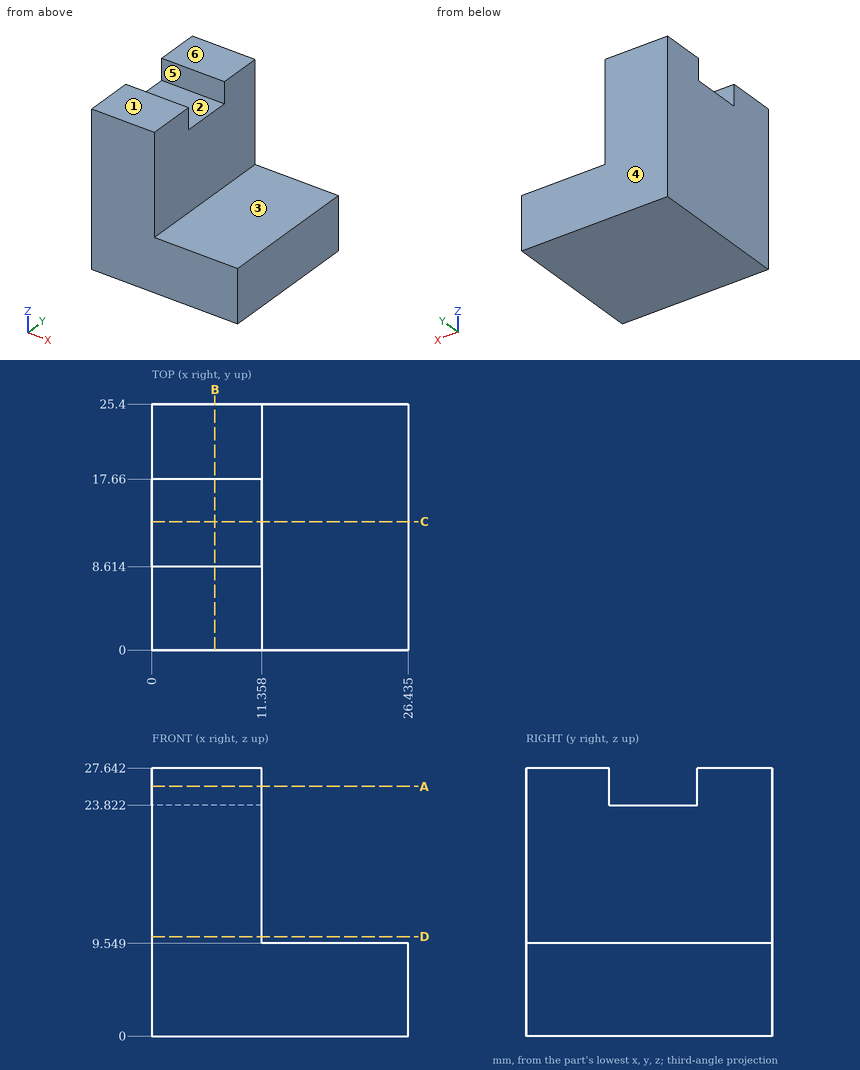
Answer from the drawing. Dimensions are ordinates in mm from the lowest x, y and z of the part. A direction names the side the tool comes from. Coordinates: 2 decimals unless noted, no trailing zeros. Order: outer loops, then holes, each group sorted by start corner. A loop starts at its lowest first (then second) coordinate and runs counter-clockwise, first axis right, second up. Notation, with made-up numbers: M 6.5,88.5 L 44.5,88.5 A26 ccw 44.5,106.5 Z; hole C 13.25,49.25 d6. An arc over 180 degrees is marked long. Put each result on its own line as item: value. Start each with the question number.
Item 1: For the marked faces 1, 2 and 3, determine the directions among +Z, -Z, +X, -X, +Y, -Y from which every point of the face is accessible in a straight line to the end or side of a thin tool.
Item 2: The mould has two halves that part along Y. Classify the marked faces 4, 5 and 6: +Y half, -Y half, draft (parallel to the pull), parting line (faces both ways), or undercut.
Item 3: Section D-D, the plane z = 10.25 is taken. Determine the outline of the cut face in (x, y).
Item 4: Section A-A, the plane z = 25.75 is taken. Determine the outline of the cut face in (x, y).
Item 5: Section B-B, the plane x = 6.5 is taken. Determine the outline of the cut face in (y, z).
Item 6: Section C-C, the plane y = 13.25 is taken. Determine the outline of the cut face in (x, z) (1 decimal).
Item 7: Consider probe 1 along Z at (x, y) = (12.25, 12.25); probe 2 along X at (y, z) = (13.25, 21); probe 3 along Z at (x, y) = (5.5, 14.5). Determine where each line is inside the solid, lowest interval first. Write a range as [from, to].
Item 8: Given pin 1 Ø2.5 at (x, y) = (7, 11.5) entering from +Z; pin 2 Ø4.5 at (x, y) = (18.5, 9.5) entering from +Z; pin 3 Ø2 at (y, z) = (3.5, 12) entering from +X, each flat-ended and moving along its own axis, determine where each tip first touches the part or whether it passes through.
Computed:
1. face 1: +Z, +X, -X, +Y, -Y
1. face 2: +Z, +X, -X
1. face 3: +Z, +X, +Y, -Y
2. face 4: +Y half
2. face 5: undercut
2. face 6: draft
3. outline: M 0,0 L 11.36,0 L 11.36,25.4 L 0,25.4 Z
4. outline: M 0,0 L 11.36,0 L 11.36,8.61 L 0,8.61 Z; M 0,17.66 L 11.36,17.66 L 11.36,25.4 L 0,25.4 Z
5. outline: M 0,0 L 25.4,0 L 25.4,27.64 L 17.66,27.64 L 17.66,23.82 L 8.61,23.82 L 8.61,27.64 L 0,27.64 Z
6. outline: M 0,0 L 26.4,0 L 26.4,9.5 L 11.4,9.5 L 11.4,23.8 L 0,23.8 Z
7. probe 1: z = [0, 9.55]
7. probe 2: x = [0, 11.36]
7. probe 3: z = [0, 23.82]
8. pin 1: stops at z = 23.82
8. pin 2: stops at z = 9.55
8. pin 3: stops at x = 11.36
